Geometry check sheet. Reference: the model listing, model coordinates, mm. Face numbers are marked on the shaded views. A direction names the side the tool comes from. Round coordinates to 2 decimals unless told otherwise and drop trailing zeros. Order: outer loops, then holes, each group sorted by start corner. A loop starts at its lowest first (then second) coordinate and runs counter-clockwise, first axis right, second up. Notation, with made-up numbers: (-8.5, 17.5) - (24.5, 17.5) arc R30 ccw to (24.5, 56.5) - close; hole circle Ø4 at (35.25, -24.5). An arc over 180 degrees is marked (long way). Return JSON: item names as keys, results as strings. Group by question number.
Q1. Sectioned sample at D-D, the plane x = -9.5. Record the cut outline in (y, z).
Q2. Draft check along X on the marked faces 1, 2, 3 and 4. Enter one of: pulls with the +X half, pulls with the -X half, needs draft (parallel to the pull), parting line crosses it, or undercut.
Q3. Sectioned sample at A-A, the plane y = 211. Record the cut outline in (x, z).
Q4. Sectioned sample at C-C, the plane z = -106. Record the cut outline in (x, y), then the cut area to 3 significant figures.
Q5. Material ranges on line 1 along X through (y, z) = (1.95, 0); line 2 along Z through (x, y) = (22, 52); line 3 along Z through (x, y) = (11.5, 8.5), recorded low to high.
Q6. Sectioned sample at B-B, the plane y = 416.5. Record the cut outline in (x, z), then the cut area to 3 significant figures.
Q7. Tool access check on the marked faces 5, 6 and 7. Record the directions out of +Z, -Z, +X, -X, +Y, -Y that give a thin tool (end or side, any length) a straight path to the whole face; none if there is none.
Q8. Gauge pin test, flat ends, axial feed: pin 1 Ø6.5 at (x, z) = (22.5, -17.5) entering from +Y; pin 2 Ø4.5 at (x, z) = (10.13, 12.37) entering from -Y; pin 3 Ø5 at (x, y) = (41.5, 327) entering from +Z. Record the tip position at first contact, or that the pin passes through.
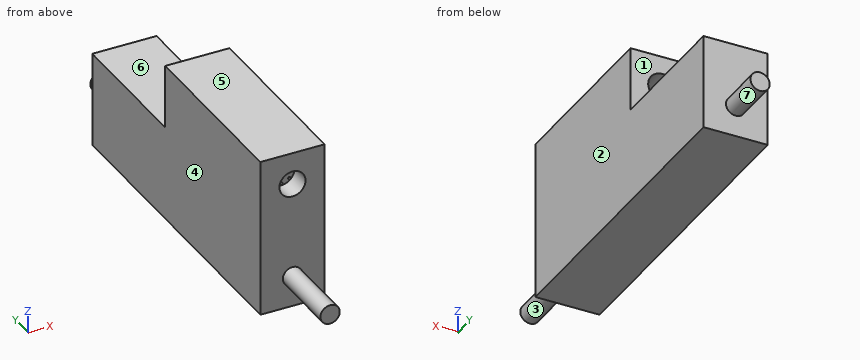
```python
from build123d import *

# Parameters (mm, degrees)
SKETCH_1_W            = 16.5
SKETCH_1_H            = 10
SKETCH_1_W_2          = 1
SKETCH_1_H_2          = 92
SKETCH_3_R            = 50
SKETCH_3_R_2          = 32.5
EXTRUDE_1_DEPTH       = 250
EXTRUDE_7_DEPTH       = 250
EXTRUDE_8_DEPTH       = 50
EXTRUDE_8_DEPTH_BACK  = 50
SKETCH_12_W           = 100
SKETCH_12_H           = 500
EXTRUDE_10_DEPTH      = 148
SKETCH_13_R           = 15
EXTRUDE_12_DEPTH      = 73
EXTRUDE_12_DEPTH_BACK = 612
SKETCH_20_W           = 80
SKETCH_20_H           = 128
SKETCH_20_R           = 15
CUT_EXTRUDE_4_DEPTH   = 470
SKETCH_20_4_W         = 80
SKETCH_20_4_H         = 128
SKETCH_20_4_R         = 15
EXTRUDE_13_DEPTH      = 10
SKETCH_1_22_W         = 6
SKETCH_1_22_H         = 10
SKETCH_22_R           = 20.32
CUT_EXTRUDE_6_DEPTH   = 33
SKETCH_23_R           = 2
CUT_EXTRUDE_7_DEPTH   = 10
SKETCH_25_R           = 14
CUT_EXTRUDE_8_DEPTH   = 3
SKETCH_26_R           = 8.75
CUT_EXTRUDE_9_DEPTH   = 4
SKETCH_27_R           = 6
CUT_EXTRUDE_10_DEPTH  = 6
CUT_EXTRUDE_12_DEPTH  = 6


with BuildPart() as part:
    # Sketch 1 → Revolve 1 (revolve)
    with BuildSketch(Plane.XY, mode=Mode.PRIVATE) as revolve_1_sk:
        Polygon((-10, 0), (0, 0), (0, 10), (0, 102), (0, 250), (-10, 250), align=None)
        with Locations((8.25, 5)):
            Rectangle(SKETCH_1_W, SKETCH_1_H)
        with Locations((36.75, 5)):
            Rectangle(SKETCH_1_W, SKETCH_1_H)
        with Locations((44.5, 56)):
            Rectangle(SKETCH_1_W_2, SKETCH_1_H_2)
        Polygon((45, 10), (45, 0), (55, 0), (55, 250), (45, 250), (45, 102), align=None)
        with Locations((0.5, 56)):
            Rectangle(SKETCH_1_W_2, SKETCH_1_H_2)
    revolve(revolve_1_sk.sketch.rotate(Axis((22.5, 0, 0), (0, 1, 0)), 270), axis=Axis((22.5, 0, 0), (0, 1, 0)))

    # Sketch 3 → Extrude 1 (add)
    with BuildSketch(Plane(origin=(0, 250, 0), x_dir=(1, 0, 0), z_dir=(0, 1, 0))):
        with Locations(Location((22.5, 0, 0), (0, 0, 270))):
            Circle(SKETCH_3_R)
        with Locations((22.5, 0)):
            Circle(SKETCH_3_R_2, mode=Mode.SUBTRACT)
    extrude(amount=-EXTRUDE_1_DEPTH)

    # Sketch 3_5 → Extrude 7 (add)
    with BuildSketch(Plane(origin=(0, 250, 0), x_dir=(1, 0, 0), z_dir=(0, 1, 0))):
        with BuildLine():
            ThreePointArc((72.5, 0), (57.855339059, -35.355339059), (22.5, -50))
            Line((22.5, -50), (72.5, -50))
            Line((72.5, -50), (72.5, 0))
        make_face()
        with BuildLine():
            ThreePointArc((22.5, -50), (-12.855339059, -35.355339059), (-27.5, 0))
            Line((-27.5, 0), (-27.5, -50))
            Line((-27.5, -50), (22.5, -50))
        make_face()
        with BuildLine():
            Line((72.5, 50), (22.5, 50))
            ThreePointArc((22.5, 50), (57.855339059, 35.355339059), (72.5, 0))
            Line((72.5, 0), (72.5, 50))
        make_face()
        with BuildLine():
            Line((-27.5, 50), (-27.5, 0))
            ThreePointArc((-27.5, 0), (-12.855339059, 35.355339059), (22.5, 50))
            Line((22.5, 50), (-27.5, 50))
        make_face()
    extrude(amount=-EXTRUDE_7_DEPTH)

    # Sketch 1_21 → Extrude 8 (add, two sides)
    with BuildSketch(Plane.XY) as extrude_8_sk:
        Polygon((16.5, 0), (0, 0), (-10, 0), (-27.5, 0), (-27.5, -33), (72.5, -33), (72.5, 0), (55, 0), (45, 0), (28.5, 0), align=None)
    extrude(amount=EXTRUDE_8_DEPTH)
    extrude(extrude_8_sk.sketch, amount=-EXTRUDE_8_DEPTH_BACK)

    # Sketch 12 → Extrude 10 (add)
    with BuildSketch(Plane(origin=(0, 0, -50), x_dir=(-1, 0, 0), z_dir=(0, 0, -1))):
        with Locations((-22.5, 217)):
            Rectangle(SKETCH_12_W, SKETCH_12_H)
    extrude(amount=EXTRUDE_10_DEPTH)

    # Sketch 13 → Extrude 12 (add, two sides)
    with BuildSketch(Plane(origin=(0, 467, 0), x_dir=(1, 0, 0), z_dir=(0, 1, 0))) as extrude_12_sk:
        with Locations(Location((22.5, 150, 0), (0, 0, 90))):
            Circle(SKETCH_13_R)
    extrude(amount=EXTRUDE_12_DEPTH)
    extrude(extrude_12_sk.sketch, amount=-EXTRUDE_12_DEPTH_BACK)

    # Sketch 20 → Cut-Extrude 4 (cut)
    with BuildSketch(Plane.XZ.offset(33)):
        with Locations((22.5, -124)):
            Rectangle(SKETCH_20_W, SKETCH_20_H)
        with Locations(Location((22.5, -150, 0), (0, 0, 270))):
            Circle(SKETCH_20_R, mode=Mode.SUBTRACT)
    extrude(amount=-CUT_EXTRUDE_4_DEPTH, mode=Mode.SUBTRACT)

    # Sketch 20_4 → Extrude 13 (add)
    with BuildSketch(Plane.XZ.offset(33)):
        with Locations((22.5, -124)):
            Rectangle(SKETCH_20_4_W, SKETCH_20_4_H)
        with Locations(Location((22.5, -150, 0), (0, 0, 270))):
            Circle(SKETCH_20_4_R, mode=Mode.SUBTRACT)
    extrude(amount=-EXTRUDE_13_DEPTH)

    # Sketch 1_22 → Revolve 2 (revolve)
    with BuildSketch(Plane.XY, mode=Mode.PRIVATE) as revolve_2_sk:
        with Locations((19.5, 5)):
            Rectangle(SKETCH_1_22_W, SKETCH_1_22_H)
    revolve(revolve_2_sk.sketch.rotate(Axis((22.5, 0, 0), (0, 1, 0)), 270), axis=Axis((22.5, 0, 0), (0, 1, 0)))

    # Sketch 22 → Cut-Extrude 6 (cut)
    with BuildSketch(Plane.XZ.offset(33)):
        with Locations(Location((22.5, 0, 0), (0, 0, 270))):
            Circle(SKETCH_22_R)
    extrude(amount=-CUT_EXTRUDE_6_DEPTH, mode=Mode.SUBTRACT)

    # Sketch 23 → Cut-Extrude 7 (cut)
    with BuildSketch(Plane.XZ):
        with Locations(Location((22.5, 17.5, 0), (0, 0, 270))):
            Circle(SKETCH_23_R)
        with Locations(Location((34.874368671, 12.374368671, 0), (0, 0, 270))):
            Circle(SKETCH_23_R)
        with Locations(Location((40, 0, 0), (0, 0, 270))):
            Circle(SKETCH_23_R)
        with Locations(Location((34.874368671, -12.374368671, 0), (0, 0, 270))):
            Circle(SKETCH_23_R)
        with Locations(Location((22.5, -17.5, 0), (0, 0, 270))):
            Circle(SKETCH_23_R)
        with Locations(Location((10.125631329, -12.374368671, 0), (0, 0, 270))):
            Circle(SKETCH_23_R)
        with Locations(Location((5, 0, 0), (0, 0, 270))):
            Circle(SKETCH_23_R)
        with Locations(Location((10.125631329, 12.374368671, 0), (0, 0, 270))):
            Circle(SKETCH_23_R)
    extrude(amount=-CUT_EXTRUDE_7_DEPTH, mode=Mode.SUBTRACT)

    # Sketch 25 → Cut-Extrude 8 (cut)
    with BuildSketch(Plane(origin=(0, 10, 0), x_dir=(1, 0, 0), z_dir=(0, 1, 0))):
        with Locations(Location((22.5, 0, 0), (0, 0, 270))):
            Circle(SKETCH_25_R)
    extrude(amount=-CUT_EXTRUDE_8_DEPTH, mode=Mode.SUBTRACT)

    # Sketch 26 → Cut-Extrude 9 (cut)
    with BuildSketch(Plane(origin=(0, 10, 0), x_dir=(1, 0, 0), z_dir=(0, 1, 0))):
        with Locations(Location((22.5, 0, 0), (0, 0, 270))):
            Circle(SKETCH_26_R)
    extrude(amount=-CUT_EXTRUDE_9_DEPTH, mode=Mode.SUBTRACT)

    # Sketch 27 → Cut-Extrude 10 (cut)
    with BuildSketch(Plane.XZ):
        with Locations(Location((22.5, 0, 0), (0, 0, 270))):
            Circle(SKETCH_27_R)
    extrude(amount=-CUT_EXTRUDE_10_DEPTH, mode=Mode.SUBTRACT)

    # Sketch 27_5 → Cut-Extrude 12 (cut)
    with BuildSketch(Plane.XZ):
        with BuildLine():
            Line((20.5, -8), (24.5, -8))
            Line((24.5, -8), (24.5, -5.656854249))
            ThreePointArc((24.5, -5.656854249), (22.5, -6), (20.5, -5.656854249))
            Line((20.5, -5.656854249), (20.5, -8))
        make_face()
    extrude(amount=-CUT_EXTRUDE_12_DEPTH, mode=Mode.SUBTRACT)


solid = part.part
```
Reply:
{
 "1": {"outline": "(-33, -198) - (467, -198) - (467, -50) - (250, -50) - (250, 50) - (-33, 50) - close; hole (-23, -188) - (437, -188) - (437, -60) - (-23, -60) - close"},
 "2": {"face 1": "needs draft", "face 2": "pulls with the +X half", "face 3": "parting line crosses it", "face 4": "pulls with the -X half"},
 "3": {"outline": "(-27.5, -198) - (72.5, -198) - (72.5, 50) - (-27.5, 50) - close; circle Ø30 at (22.5, -150); hole (-17.5, -188) - (62.5, -188) - (62.5, -60) - (-17.5, -60) - close; hole circle Ø45 at (22.5, 0)"},
 "4": {"outline": "(-27.5, -33) - (72.5, -33) - (72.5, 467) - (-27.5, 467) - close; hole (-17.5, -23) - (62.5, -23) - (62.5, 437) - (-17.5, 437) - close", "area": "13,200 mm^2"},
 "5": {"line 1": "-27.5 to 3, 7 to 16.5, 28.5 to 38, 42 to 72.5", "line 2": "-198 to -188, -164.99 to -135.01, -60 to -21.49, 21.49 to 50", "line 3": "-198 to -188, -160.2 to -139.8, -60 to -13.83, -10.92 to -8.66, 8.66 to 10.92, 13.83 to 50"},
 "6": {"outline": "(-27.5, -198) - (72.5, -198) - (72.5, -50) - (-27.5, -50) - close; circle Ø30 at (22.5, -150); hole (-17.5, -188) - (62.5, -188) - (62.5, -60) - (-17.5, -60) - close", "area": "5,270 mm^2"},
 "7": {"face 5": "+Z, +X, -X, +Y, -Y", "face 6": "+Z, +X, -X, +Y", "face 7": "+Y"},
 "8": {"pin 1": "y = 10", "pin 2": "y = 0", "pin 3": "z = -50"}
}
